Solid Edge part; units mm, degrees
sketch "Sketch1" plane through (0, 0, 0) normal (0, 0, 1) x (1, 0, 0)
  line L0 (30, 0) -> (30, 90)
  line L1 (30, 90) -> (0, 90)
  line L2 (0, 90) -> (0, 0)
  line L3 (0, 0) -> (30, 0)
extrude "Protrusion1" add sketch "Sketch1" along normal blind 45
sketch "Sketch2" plane through (15, 45, 45) normal (0, 0, 1) x (1, 0, 0)
  line L0 (-15, 45) -> (33, 45)
  line L1 (33, 45) -> (33, -45)
  line L2 (33, -45) -> (-15, -45)
  line L3 (-15, -45) -> (-15, 45)
extrude "ExtrudedProtrusion_2" add sketch "Sketch2" along normal blind 12
sketch "Sketch3" plane through (24, 45, 57) normal (0, 0, 1) x (1, 0, 0)
  line L0 (-24, -45) -> (6, -45)
  line L1 (6, -45) -> (6, 45)
  line L2 (6, 45) -> (-24, 45)
  line L3 (-24, 45) -> (-24, -45)
extrude "ExtrudedProtrusion_3" add sketch "Sketch3" along normal blind 10
sketch "Sketch4" plane through (0, 45, 33.5) normal (-1, 0, 0) x (0, 0, 1)
  line L0 (69.5, 45) -> (69.5, 0)
  line L1 (69.5, 0) -> (33.5, -45)
  line L2 (33.5, 45) -> (33.5, -45)
  line L3 (33.5, 45) -> (69.5, 45)
extrude "ExtrudedProtrusion_5" add sketch "Sketch4" against normal blind 50
sketch "Sketch5" plane through (50, 45, 85) normal (1, 0, 0) x (0, 1, 0)
  line L0 (45, -18) -> (45, -4)
  line L1 (45, -4) -> (-25.0048, -2.0039)
  line L2 (-25.0048, -2.0039) -> (-45, -18)
  line L3 (-45, -18) -> (45, -18)
extrude "ExtrudedCutout_6" cut sketch "Sketch5" against normal blind 20
sketch "Sketch6" plane through (15, 45, 0) normal (0, 0, -1) x (0, 1, 0)
  line L0 (-25.2561, -7) -> (-25.2561, 5)
  line L1 (-25.2561, 5) -> (-34.6265, 5)
  line L2 (-34.6265, 5) -> (-34.6265, -7)
  line L3 (-34.6265, -7) -> (-25.2561, -7)
extrude "ExtrudedCutout_7" cut sketch "Sketch6" against normal blind 588.5853
sketch "Sketch7" plane through (25, 67.5, 103) normal (0, 0, 1) x (0, 1, 0)
  line L0 (22.5, 25) -> (-17.5, 25)
  line L1 (-17.5, 25) -> (-17.5, 7)
  line L2 (-17.5, 7) -> (22.5, 7)
  line L3 (22.5, 7) -> (22.5, 25)
extrude "ExtrudedCutout_8" cut sketch "Sketch7" against normal blind 143.8541
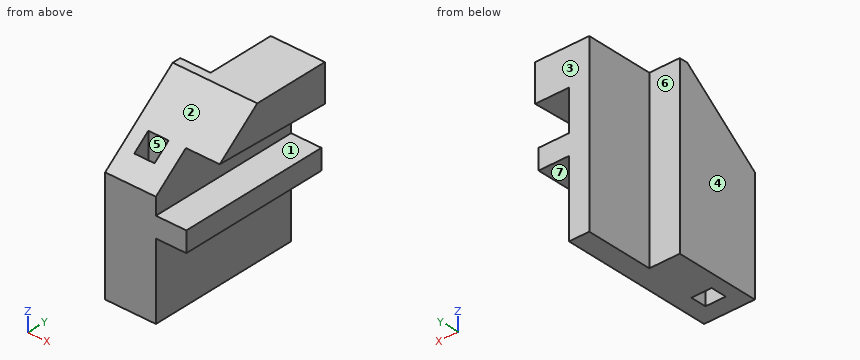
Input: part model. Units: mm. Frame: model coordinates. Face numbers are marked on the shaded views. A direction names the side the tool comes from. Round coordinates to 2 decimals unless told otherwise and drop trailing zeros. Loops run counter-clockwise (first coordinate to the right, second up) from the corner with the lowest first, then second, coordinate; pieces in that order, holes last. Notation, with made-up numbers: (75.5, -9) -> (120.5, -9) arc R21 cw to (120.5, 27) -> close; hole circle Ø10 at (80.25, 42.5). An arc over 180 degrees is marked (long way). Write each question's results on one line, items separated by ' | '.
1. Section A-A (x = 38.5). Return loops of the section in (y, z).
Geometry results:
outline: (0, 45) -> (90, 45) -> (90, 57) -> (0, 57) -> close; (20, 83) -> (90, 81) -> (90, 103) -> (45, 103) -> close
2. Set-up query: the marked faces 4, 5, 6 and 7. Return all of +Z, -Z, +X, -X, +Y, -Y with unobstructed straight access to the full face (end or side cutting, diameter ignored); none if empty.
Geometry results:
face 4: +Z, -Z, -X, +Y, -Y | face 5: +Z, -Z | face 6: +Z, -Z, -X, +Y | face 7: -Z, +X, +Y, -Y
3. Section B-B (y = 18). Return loops of the section in (x, z), and give its area (3 significant figures).
Geometry results:
outline: (0, 0) -> (8, 0) -> (8, 81.4) -> (0, 81.4) -> close; (20, 0) -> (30, 0) -> (30, 45) -> (48, 45) -> (48, 57) -> (30, 57) -> (30, 81.4) -> (20, 81.4) -> close | area: 1,680 mm2
4. Mould query, pull axis Z, two halves, no side actions, for the marked faces 1, 2 and 3. Classes: +Z half, -Z half, draft (parallel to the pull), parting line (faces both ways), or undercut.
Geometry results:
face 1: undercut | face 2: +Z half | face 3: draft
5. Section C-C (z = 33). Return loops of the section in (x, y).
Geometry results:
outline: (0, 0) -> (30, 0) -> (30, 90) -> (18, 90) -> (18, 50) -> (0, 50) -> close; hole (8, 10.37) -> (20, 10.37) -> (20, 19.74) -> (8, 19.74) -> close
6. Section D-D (x = 21.5). Return loops of the section in (y, z).
Geometry results:
outline: (0, 0) -> (90, 0) -> (90, 103) -> (45, 103) -> (0, 67) -> close
7. First-contact query: P1, Ø10.5, axis at y = 13.5, z = 43.5, coming from the +X side; P2, Ø6, axis at x = 13, z = 19.5, coming from the +Y side; P3, Ø6, axis at x = 12, z = 81, coming from the -Y side. Flat tips, straight axial feed; report the tip coordinate or a pass-through.
Geometry results:
P1: x = 48 | P2: y = 50 | P3: y = 19.74
8. Ray query, line 1 (Y direction, x = 18.5, z = 55.5); line 2 (X direction, y = 12, z = 10); line 3 (X direction, y = 49, z = 79.5). Return the intervals inside material, ascending. Write a range as from..to.
Geometry results:
line 1: 0..10.37, 19.74..90 | line 2: 0..8, 20..30 | line 3: 0..30
